Could you check a few things on this drawing? It's one solid part, dimensions in mm from its lowest x, y, z. A direction names the side the tool comes from. Give positions to 0.01 mm unless a question says otherwise; leave off trailing zeros. Loops run counter-clockwise (first coordinate to the right, second up) from the corner with the lowest first, then second, coordinate; pieces in that order, holes last.
1. Imagine slicing it at C-C (z = 7.75). List the corners of the cut face in (x, y) for me.
2. Imagine slicing it at A-A (x = 5). List the corners of the cut face in (y, z) for me.
3. Imagine slicing it at B-B (z = 5). List the corners of the cut face in (x, y) for me.
4. I need wall thicknesses on line 1 along Y through (x, z) = (3.5, 2.25); line 2 along X through (y, z) = (7.25, 1.5); line 3 along Z through (x, y) = (8.5, 12.25). Which ranges of each line are inside material? Lowest first, please.
5. Imagine slicing it at D-D (y = 10.75). List the corners of the cut face in (x, z) for me.
6. For P1, Ø3, axis at x = 8, z = 4.5, coming from the -Y side; P2, Ø2, axis at y = 9.5, z = 7.5, coming from the -X side; P3, Ø1.5, axis at y = 4, z = 2, coming from the -X side; P4, Ø1.5, axis at y = 10, z = 5.5, coming from the +X side, each with a flat end and sliding along its axis, tell me the tip position at first contact or that it passes through.
7. For the marked faces 1 and 2, which set-ups out of +Z, -Z, +X, -X, +Y, -Y let a thin tool reach every point of the face, with its end or its side?
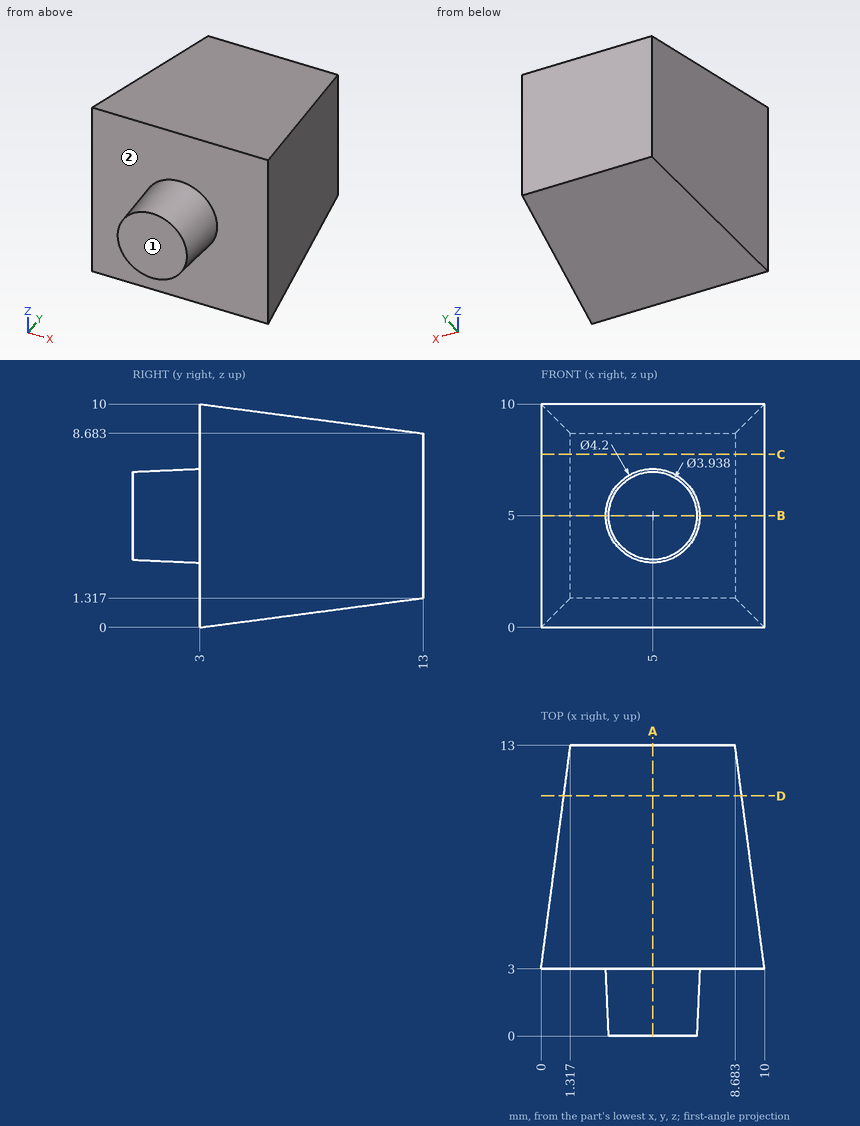
Derived:
1. outline: (0, 3) - (10, 3) - (8.68, 13) - (1.32, 13) - close
2. outline: (0, 3.03) - (3, 2.9) - (3, 0) - (13, 1.32) - (13, 8.68) - (3, 10) - (3, 7.1) - (0, 6.97) - close
3. outline: (0, 3) - (2.9, 3) - (3.03, 0) - (6.97, 0) - (7.1, 3) - (10, 3) - (8.68, 13) - (1.32, 13) - close
4. line 1: y = 3 to 13
4. line 2: x = 0.56 to 9.44
4. line 3: z = 1.22 to 8.78
5. outline: (1.02, 1.02) - (8.98, 1.02) - (8.98, 8.98) - (1.02, 8.98) - close
6. P1: stops at y = 0
6. P2: stops at x = 0.72
6. P3: stops at x = 0.03
6. P4: stops at x = 9.18
7. face 1: +Z, -Z, +X, -X, -Y
7. face 2: -Y
